Read the model definition and answer for the solid it produces. Units are mm, in the model's axes. Coordinates: 2 decimals unless noted, no trailing zeros. Write each loop counter-clockwise with the first axis right and the second up, starting at its lowest first coordinate (ties: lowest second). Pieces come first, ordered by that corner, then holes.
1) The part is cut by section B-B (x = 35.5). Determine the outline of the cut face in (y, z), then the cut area to 3 significant figures.
2) The part is cut by section D-D (z = 3.25). Determine the outline of the cut face in (x, y).
3) The part is cut by section A-A (z = 15). Determine the outline of the cut face in (x, y).
4) Each of these flat-tipped pins is pushed along its axis until it touches: pin 1 Ø4 at (y, z) = (-3, 18.5) entering from +X; pin 2 Ø3 at (x, y) = (40, -3) entering from +Z. Where does it stop, or does it pass through?
5) Determine the mould class of faces 1 (the face through (18, -6, 30)), 2 (the face through (50, -6, 15)), 3 (the face through (41.743, -5.916, 15.297)), 4 (the face through (25, -12, 15)) for opening direction Z: +Z half, -Z half, draft (parallel to the pull), parting line (faces both ways), or undercut.
6) The part is cut by section C-C (y = -6.25). Determine the outline of the cut face in (x, z).
7) Find the intervals of material crossed by line 1 (Z direction, x = 35, y = -3); line 2 (X direction, y = -2.25, z = 18.5); line 3 (X direction, y = -4.75, z = 13.75), in increasing order.
from build123d import *

# Parameters (mm, degrees)
F1_DEPTH = 12
F3_D     = 13.5


with BuildPart() as f1:
    # F0 (on Front) → F1 (new body)
    with BuildSketch(Plane.XZ):
        with BuildLine():
            Line((0, 30), (0, 0))
            Line((0, 0), (35, 0))
            ThreePointArc((35, 0), (45.6066017178, 4.3933982822), (50, 15))
            ThreePointArc((50, 15), (45.6066017178, 25.6066017178), (35, 30))
            Line((35, 30), (0, 30))
        make_face()
    extrude(amount=F1_DEPTH)

    # F3 (through all)
    with Locations(Plane.XZ.offset(12)):
        with Locations((35, 15)):
            Hole(F3_D / 2)


solid = f1.part
Reported:
1. outline: (-12, 0.01) - (0, 0.01) - (0, 8.27) - (-12, 8.27) - close; (-12, 21.73) - (0, 21.73) - (0, 29.99) - (-12, 29.99) - close
1. area: 198 mm2
2. outline: (0, -12) - (44.32, -12) - (44.32, 0) - (0, 0) - close
3. outline: (0, -12) - (28.25, -12) - (28.25, 0) - (0, 0) - close; (41.75, -12) - (50, -12) - (50, 0) - (41.75, 0) - close
4. pin 1: stops at x = 49.92
4. pin 2: stops at z = 29.59
5. face 1: +Z half
5. face 2: parting line
5. face 3: undercut
5. face 4: draft
6. outline: (0, 0) - (35, 0) arc R15 ccw to (35, 30) - (0, 30) - close; hole circle Ø13.5 at (35, 15)
7. line 1: z = 0 to 8.25, 21.75 to 30
7. line 2: x = 0 to 29.23, 40.77 to 49.59
7. line 3: x = 0 to 28.37, 41.63 to 49.95
